Design review of the part shown in the three views and the two pictorial views. Dimensions are in mm from the part's minimum x, y and z. A direction names the side the tool comes from. Round coordinates to 2 decimals unless told otherwise and drop trailing zeros. Loops run counter-clockwise (first coordinate to the right, second up) from the corner with the lowest first, then second, coordinate; pieces in that order, holes last. Notation, with made-up numbers: (65.25, 59) -> (81.25, 59) arc R32 cw to (81.25, 86) -> close; hole circle Ø8 at (-8, -38.5). An arc over 180 degrees is marked (long way). One line per question, with ' | ' between items. Start each with the question number.
1. Consider section D-D (y = 4.6). Write out the cut boundary in (x, z), and give its area (3 significant figures).
2. For the marked faces 1 and 2, list the 3-axis set-ups (+Z, -Z, +X, -X, +Y, -Y) from which the entire face can be reached by the end or side of a thin tool; tool diameter is ignored.
3. Consider section A-A (x = 2.5). Write out the cut boundary in (y, z).
4. Draft analysis for pull direction X (two halves, no side actions). For the marked faces 3, 4 and 5, state which applies: pulls with the +X half, pulls with the -X half, needs draft (parallel to the pull), parting line crosses it, or undercut.
5. Consider section B-B (y = 1.95). Write out the cut boundary in (x, z).
6. Consider section C-C (z = 8.25). Write out the cut boundary in (x, y).
7. For pin 1 Ø1.5 at (x, y) = (3, 2.5) entering from -Z; pin 2 Ø1 at (y, z) = (4, 2) entering from -X, all flat-tipped, find the tip position at first contact; note any pin that passes through.
8. Wall thickness on line 1 along Y through (x, z) = (2.5, 6.5); line 2 along Y through (x, z) = (1.75, 0.75); line 3 along X through (y, z) = (1.75, 8.5): over which ranges is each line inside the solid? List them lowest first.
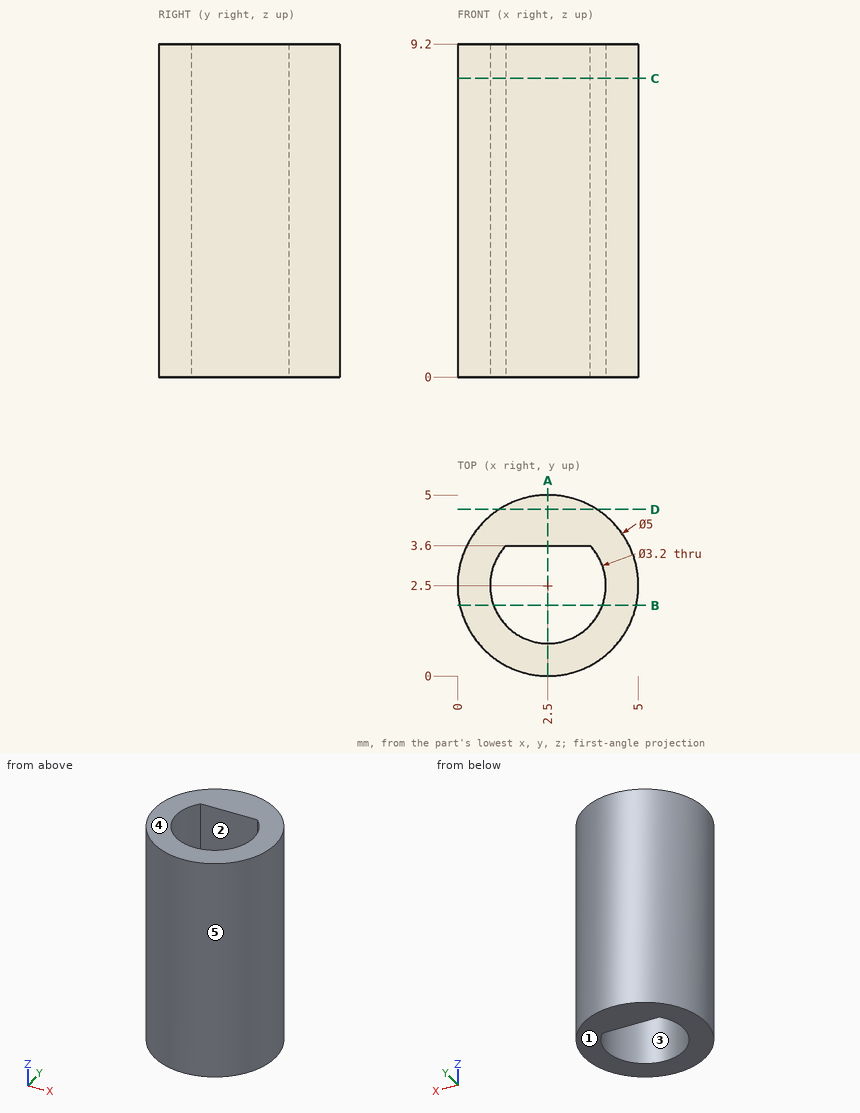
Answer block:
1) outline: (1.14, 0) -> (3.86, 0) -> (3.86, 9.2) -> (1.14, 9.2) -> close | area: 25.0 mm2
2) face 1: -Z, +X, -X, +Y, -Y | face 2: +Z, -Z
3) outline: (0, 0) -> (0.9, 0) -> (0.9, 9.2) -> (0, 9.2) -> close; (3.6, 0) -> (5, 0) -> (5, 9.2) -> (3.6, 9.2) -> close
4) face 3: undercut | face 4: needs draft | face 5: parting line crosses it
5) outline: (0.06, 0) -> (1, 0) -> (1, 9.2) -> (0.06, 9.2) -> close; (4, 0) -> (4.94, 0) -> (4.94, 9.2) -> (4, 9.2) -> close
6) outline: circle Ø5 at (2.5, 2.5); hole (1.34, 3.6) arc R1.6 ccw (long way) to (3.66, 3.6) -> close
7) pin 1: passes through | pin 2: stops at x = 0.21
8) line 1: y = 0 to 0.9, 3.6 to 5 | line 2: y = 0.12 to 1.09, 3.6 to 4.88 | line 3: x = 0.12 to 1.09, 3.91 to 4.88
